Source: three-view drawing plus pictorial views. Frame: mm from the lowest corner of the part. Give positions to 0.01 mm unless a question says otherwise; leave off trailing zeros. Loops run counter-clockwise (first coordinate to the right, second up) from the corner with the lowest first, then second, coordinate; pieces in that order, holes last. Notation, with made-up numbers: (30.5, -28.5) - (46.5, -28.5) arc R30 cw to (46.5, -1.5) - close; hole circle Ø11 at (2.5, 46.25). An arc over 180 degrees is marked (long way). Answer as a JSON object with one key per item and string values. Group by question number.
(1) Section query B-B (y = 27). Return loops of the section in (x, z), plus the area to 3 significant figures.
(2) Section query C-C (y = 15). Return loops of the section in (x, z).
(3) Material intervals for L1, parallel to Y at x = 130.5, z = 2.5; L2, parallel to X at y = 33.5, z = 0.6; L3, parallel to X at y = 31, z = 3.1, sorted ascending.
(4) Section query D-D (y = 36). Return loops of the section in (x, z).
(5) Pin query (flat end, axial travel): P1, Ø1.5, axis at y = 27, z = 2.5, coming from the -X side; P2, Ø0.8, axis at y = 18, z = 2.5, coming from the +X side. Return the tip coordinate at first contact, or that it passes through.
(6) Section query A-A (x = 68.5). Return loops of the section in (y, z), plus the area to 3 significant figures.
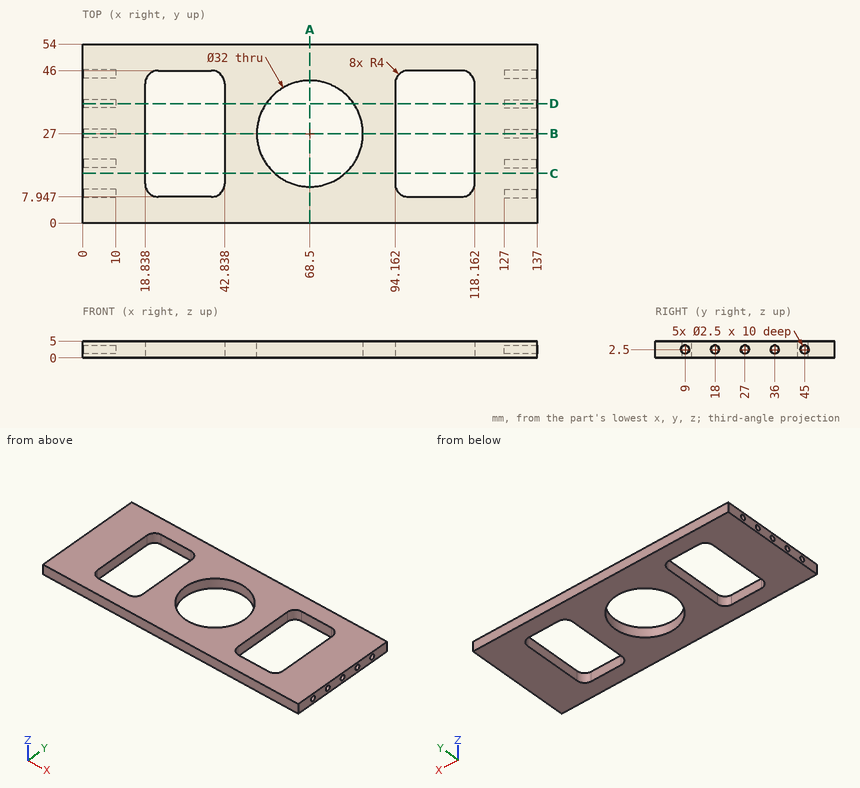
Recorded:
{
 "1": {"outline": "(0, 0) - (18.84, 0) - (18.84, 5) - (0, 5) - (0, 3.75) - (10, 3.75) - (10, 1.25) - (0, 1.25) - close; (42.84, 0) - (52.5, 0) - (52.5, 5) - (42.84, 5) - close; (84.5, 0) - (94.16, 0) - (94.16, 5) - (84.5, 5) - close; (118.16, 0) - (137, 0) - (137, 1.25) - (127, 1.25) - (127, 3.75) - (137, 3.75) - (137, 5) - (118.16, 5) - close", "area": "235 mm^2"},
 "2": {"outline": "(0, 0) - (18.84, 0) - (18.84, 5) - (0, 5) - close; (42.84, 0) - (57.92, 0) - (57.92, 5) - (42.84, 5) - close; (79.08, 0) - (94.16, 0) - (94.16, 5) - (79.08, 5) - close; (118.16, 0) - (137, 0) - (137, 5) - (118.16, 5) - close"},
 "3": {"L1": "y = 0 to 7.75, 10.25 to 16.75, 19.25 to 25.75, 28.25 to 34.75, 37.25 to 43.75, 46.25 to 54", "L2": "x = 0 to 18.84, 42.84 to 53.88, 83.12 to 94.16, 118.16 to 137", "L3": "x = 0 to 18.84, 42.84 to 53.01, 83.99 to 94.16, 118.16 to 137"},
 "4": {"outline": "(0, 0) - (18.84, 0) - (18.84, 5) - (0, 5) - (0, 3.75) - (10, 3.75) - (10, 1.25) - (0, 1.25) - close; (42.84, 0) - (55.27, 0) - (55.27, 5) - (42.84, 5) - close; (81.73, 0) - (94.16, 0) - (94.16, 5) - (81.73, 5) - close; (118.16, 0) - (137, 0) - (137, 1.25) - (127, 1.25) - (127, 3.75) - (137, 3.75) - (137, 5) - (118.16, 5) - close"},
 "5": {"P1": "stops at x = 10", "P2": "stops at x = 127"},
 "6": {"outline": "(0, 0) - (11, 0) - (11, 5) - (0, 5) - close; (43, 0) - (54, 0) - (54, 5) - (43, 5) - close", "area": "110 mm^2"}
}
